```python
from build123d import *

# Parameters (mm, degrees)
F2_R     = 5.08
F3_R     = 92.6849433369
F4_DEPTH = 63.5


with BuildPart() as f1:
    # F0 (on Top) → F1 (revolve)
    with BuildSketch(Plane.XY):
        with BuildLine():
            add(Edge.make_bspline(
                [(0, 55.555421859), (24.8840127034, 59.7938904443), (73.3911612301, 68.0560637377), (37.2265693027, 30.0505371245), (33.7679755354, 9.4028379089)],
                knots=[0, 0, 0, 0, 0.2464873133, 0.4804850752, 0.4804850752, 0.4804850752, 0.4804850752], degree=3))
            Line((0, 55.555421859), (0, 11.5997837856))
            add(Edge.make_bspline(
                [(0, 11.5997837856), (11.795305595, 10.8945052523), (23.5906111899, 10.189226719), (33.7679755342, 9.4028379092)],
                knots=[0, 0, 0, 0, 0.1849290506, 0.1849290506, 0.1849290506, 0.1849290506], degree=3))
        make_face()
        with BuildLine():
            add(Edge.make_bspline(
                [(0, 11.5997837856), (11.795305595, 10.8945052523), (23.5906111899, 10.189226719), (33.7679755342, 9.4028379092)],
                knots=[0, 0, 0, 0, 0.1849290506, 0.1849290506, 0.1849290506, 0.1849290506], degree=3))
            Line((0, 11.5997837856), (0, -9.434199892))
            add(Edge.make_bspline(
                [(33.6469726445, -3.8624940343), (23.4971770517, -5.666295762), (11.7485885258, -7.550247827), (0, -9.434199892)],
                knots=[0.8153025479, 0.8153025479, 0.8153025479, 0.8153025479, 1, 1, 1, 1], degree=3))
            add(Edge.make_bspline(
                [(33.7679755354, 9.4028379089), (33.4862186228, 7.720757741), (32.9996571351, 3.3265179559), (33.2676792764, -1.1309282402), (33.6469726587, -3.8624940329)],
                knots=[0.4804850752, 0.4804850752, 0.4804850752, 0.4804850752, 0.4995478769, 0.5298676984, 0.5298676984, 0.5298676984, 0.5298676984], degree=3))
        make_face()
        with BuildLine():
            add(Edge.make_bspline(
                [(33.7679755342, 9.4028379092), (50.9954766221, 8.071696209), (76.3517739328, 4.9230972696), (51.0859067291, -0.7632809374), (33.6469726445, -3.8624940343)],
                knots=[0.1849290506, 0.1849290506, 0.1849290506, 0.1849290506, 0.4979634781, 0.8153025479, 0.8153025479, 0.8153025479, 0.8153025479], degree=3))
            add(Edge.make_bspline(
                [(33.7679755354, 9.4028379089), (33.4862186228, 7.720757741), (32.9996571351, 3.3265179559), (33.2676792764, -1.1309282402), (33.6469726587, -3.8624940329)],
                knots=[0.4804850752, 0.4804850752, 0.4804850752, 0.4804850752, 0.4995478769, 0.5298676984, 0.5298676984, 0.5298676984, 0.5298676984], degree=3))
        make_face()
        with BuildLine():
            add(Edge.make_bspline(
                [(33.6469726445, -3.8624940343), (23.4971770517, -5.666295762), (11.7485885258, -7.550247827), (0, -9.434199892)],
                knots=[0.8153025479, 0.8153025479, 0.8153025479, 0.8153025479, 1, 1, 1, 1], degree=3))
            Line((0, -9.434199892), (0, -47.1875108778))
            add(Edge.make_bspline(
                [(33.6469726587, -3.8624940329), (36.5407583141, -24.7027361152), (67.8249934472, -66.4419011922), (22.847107765, -53.6734257022), (0, -47.1875108778)],
                knots=[0.5298676984, 0.5298676984, 0.5298676984, 0.5298676984, 0.7611901228, 1, 1, 1, 1], degree=3))
        make_face()
    revolve(axis=Axis((0, -0.2655424178, 0), (0, -1, 0)))

    # F2
    f2_edges = [f1.edges().sort_by_distance(p)[0] for p in [
        (-33.767976, 9.402838, 0),
        (63.595971, 3.942528, 0),
        (51.504613, 57.585198, 0),
        (-33.646973, -3.862494, 0),
        (48.940167, -52.384771, 0),
    ]]
    fillet(f2_edges, radius=F2_R)


with BuildPart() as f4:
    # F3 (on Front) → F4 (new body, symmetric)
    with BuildSketch(Plane.XZ):
        Circle(F3_R)
    extrude(amount=F4_DEPTH, both=True)

    # F5: cut F1
    add(f1.part, mode=Mode.SUBTRACT)


solid = f4.part
```
The model under review builds one solid part; all positions refer to its coordinate system, in mm. Coordinates: 2 decimals unless noted, no trailing zeros. Write each loop counter-clockwise with the first axis right and the second up, starting at its lowest first coordinate (ties: lowest second). Pieces come first, ordered by that corner, then holes. Notation, with made-up numbers: (56.25, 3) - (114.25, 3) arc R15 cw to (114.25, 20) - close; hole circle Ø11 at (-28, 32.5). An arc over 180 degrees is marked (long way). Answer in a Markdown table with one row per item. Add a question column.
Q1. To check wall thickness, follow line 1 along X through (y, z) = (26, 23.5); line 2 along Y through (x, z) = (1, 31.5); line 3 along Y through (x, z) = (-36, 18.5). State the ranges of each line that lie inside material, in increasing order. Write a range as from..to.
Q2. Clearance check with flat-ended pins moving along their axes: pin 1 (6 mm diameter, centred on x = 43.5, y = -47.5, fed in from +Z); pin 2 (5 mm diameter, centred on x = 6.5, y = 14, fed in from +Z); pin 3 (5 mm diameter, centred on y = -19.5, z = 35, fed in from +X). State where each tip first meets the part, or that it passes through.
Q3. Consider section A-A on x = 75. Give the boundary of the cut face in (y, z), then the cut area to 3 significant figures.
Answers below:
| question | item | result |
|---|---|---|
| 1 | line 1 | -89.66..-31.41, 31.41..89.66 |
| 1 | line 2 | -63.5..-55.11, 60.16..63.5 |
| 1 | line 3 | -63.5..-56, -26.34..-2.61, 8.85..28.6, 60.55..63.5 |
| 2 | pin 1 | z = 83.37 |
| 2 | pin 2 | z = 92.6 |
| 2 | pin 3 | x = 86.8 |
| 3 | outline | (-63.5, -54.46) - (63.5, -54.46) - (63.5, 54.46) - (-63.5, 54.46) - close |
| 3 | area | 13,800 mm² |
